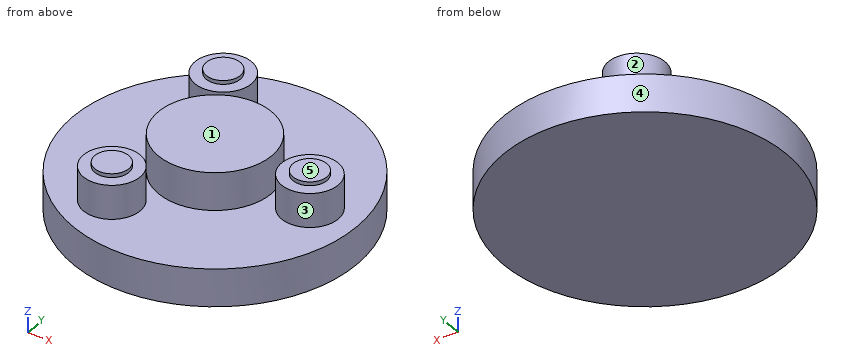
from build123d import *

# Parameters (mm, degrees)
SKETCH_1_R  = 37.5
PAD_1_DEPTH = 10
SKETCH_2_R  = 15
PAD_2_DEPTH = 10
SKETCH_3_R  = 4.5
PAD_3_DEPTH = 10
SKETCH_4_R  = 7.5
PAD_4_DEPTH = 9
SKETCH_5_R  = 4.5
PAD_5_DEPTH = 10
SKETCH_6_R  = 7.5
PAD_6_DEPTH = 9
SKETCH_7_R  = 4.5
PAD_7_DEPTH = 10
SKETCH_8_R  = 7.5
PAD_8_DEPTH = 9


with BuildPart() as part:
    # Sketch_1 → Pad_1 (new body)
    with BuildSketch(Plane.XY):
        Circle(SKETCH_1_R)
    extrude(amount=PAD_1_DEPTH)

    # Sketch_2 (on Face3 of Pad_1) → Pad_2 (join)
    with BuildSketch(Plane.XY.offset(10)):
        Circle(SKETCH_2_R)
    extrude(amount=PAD_2_DEPTH)

    # Sketch_3 (on Face3 of Pad_2) → Pad_3 (join)
    with BuildSketch(Plane.XY.offset(10)):
        with Locations((25, 0)):
            Circle(SKETCH_3_R)
    extrude(amount=PAD_3_DEPTH)

    # Sketch_4 (on Face3 of Pad_3) → Pad_4 (join)
    with BuildSketch(Plane.XY.offset(10)):
        with Locations((25, 0)):
            Circle(SKETCH_4_R)
    extrude(amount=PAD_4_DEPTH)

    # Sketch_5 (on Face3 of Pad_4) → Pad_5 (join)
    with BuildSketch(Plane.XY.offset(10)):
        with Locations((-12.5, 21.650635)):
            Circle(SKETCH_5_R)
    extrude(amount=PAD_5_DEPTH)

    # Sketch_6 (on Face3 of Pad_5) → Pad_6 (join)
    with BuildSketch(Plane.XY.offset(10)):
        with Locations((-12.5, 21.650635)):
            Circle(SKETCH_6_R)
    extrude(amount=PAD_6_DEPTH)

    # Sketch_7 (on Face3 of Pad_6) → Pad_7 (join)
    with BuildSketch(Plane.XY.offset(10)):
        with Locations((-12.5, -21.650635)):
            Circle(SKETCH_7_R)
    extrude(amount=PAD_7_DEPTH)

    # Sketch_8 (on Face3 of Pad_7) → Pad_8 (join)
    with BuildSketch(Plane.XY.offset(10)):
        with Locations((-12.5, -21.650635)):
            Circle(SKETCH_8_R)
    extrude(amount=PAD_8_DEPTH)


solid = part.part
Model file for the job. Use its own axes, mm. Face numbers are marked on the shaded views. A direction names the side the tool comes from. Give positions to 0.01 mm unless a question says otherwise; leave off trailing zeros. Loops run counter-clockwise (first coordinate to the right, second up) from the corner with the lowest first, then second, coordinate; pieces in that order, holes last.
1) Pull direction X, two halves, no side cores. Call the marked faces 3, 4 and 5: +X half, -X half, draft (parallel to the pull), parting line (faces both ways), or undercut.
2) Flat gauge pins, fed straight in: pin 1 Ø12 at (x, y) = (7, 30) entering from -Z; pin 2 Ø6 at (x, z) = (-0.5, 10) entering from +Y; pin 3 Ø10 at (y, z) = (9.5, 14) entering from +X; pin 4 Ø2 at (y, z) = (-20, 4) entering from -X. Where does each tip first touch, or does it go through?
3) Saw through at D-D (z = 8). Write the cut outline in (x, y).
4) Wall check: line 1 (Y direction, x = 25, z = 17.25); line 2 (Z direction, x = -32, y = 5.5); line 3 (X direction, y = -1, z = 5.75). Give the ranges that are in metal, low to high.
5) Saw through at B-B (x = 0). Write the cut outline in (y, z), plus the area to 3 significant figures.
6) Saw through at C-C (z = 13). Write the cut outline in (x, y), plus the area to 3 significant figures.
7) Saw through at A-A (y = 0). Write the cut outline in (x, z), plus the area to 3 significant figures.
8) Tool access for the marked faces 1 and 2: list every direction of +Z, -Z, +X, -X, +Y, -Y with a clear straight run to the whole face (end or side of a thin tool).
Answer block:
1. face 3: undercut
1. face 4: parting line
1. face 5: draft
2. pin 1: stops at z = 0
2. pin 2: stops at y = 37.5
2. pin 3: stops at x = 36.93
2. pin 4: stops at x = -32.33
3. outline: circle Ø75 at (0, 0)
4. line 1: y = -7.5 to 7.5
4. line 2: z = 0 to 10
4. line 3: x = -37.49 to 37.49
5. outline: (-37.5, 0) - (37.5, 0) - (37.5, 10) - (15, 10) - (15, 20) - (-15, 20) - (-15, 10) - (-37.5, 10) - close
5. area: 1,050 mm2
6. outline: circle Ø15 at (-12.5, -21.65); circle Ø15 at (-12.5, 21.65); circle Ø30 at (0, 0); circle Ø15 at (25, 0)
6. area: 1,240 mm2
7. outline: (-37.5, 0) - (37.5, 0) - (37.5, 10) - (32.5, 10) - (32.5, 19) - (29.5, 19) - (29.5, 20) - (20.5, 20) - (20.5, 19) - (17.5, 19) - (17.5, 10) - (15, 10) - (15, 20) - (-15, 20) - (-15, 10) - (-37.5, 10) - close
7. area: 1,190 mm2
8. face 1: +Z, +X, -X, +Y, -Y
8. face 2: +Z
